```python
from build123d import *

# Parameters (mm, degrees)
SKETCH1_W           = 140
SKETCH1_H           = 93.753760253
BOSS_EXTRUDE1_DEPTH = 1.5
SKETCH2_R           = 1.6
CUT_EXTRUDE1_DEPTH  = 1.5
SKETCH3_R           = 2.737611944
SKETCH3_R_2         = 1.237611944
BOSS_EXTRUDE2_DEPTH = 8
SKETCH4_R           = 1.3
SKETCH4_R_2         = 1.35
SKETCH4_R_3         = 1.5875
CUT_EXTRUDE2_DEPTH  = 8


with BuildPart() as part:
    # Sketch1 → Boss-Extrude1 (new body)
    with BuildSketch(Plane.XY):
        with Locations((102, 196.095777869)):
            Rectangle(SKETCH1_W, SKETCH1_H)
    extrude(amount=BOSS_EXTRUDE1_DEPTH)

    # Sketch2 → Cut-Extrude1 (cut)
    with BuildSketch(Plane.XY.offset(1.5)):
        with Locations((47.04400772, 240.027868216)):
            Circle(SKETCH2_R)
        with Locations((162.04400772, 240.027868216)):
            Circle(SKETCH2_R)
    extrude(amount=-CUT_EXTRUDE1_DEPTH, mode=Mode.SUBTRACT)

    # Sketch3 → Boss-Extrude2 (add)
    # profile 1 of 2: a face of its own
    with BuildSketch(Plane.XY.offset(1.5)):
        with Locations((47.04400772, 156.027868216)):
            Circle(SKETCH3_R)
        with Locations((47.04400772, 156.027868216)):
            Circle(SKETCH3_R_2, mode=Mode.SUBTRACT)
    # profile 2 of 2: a face of its own
    with BuildSketch(Plane.XY.offset(1.5)):
        with Locations((162.04400772, 156.027868216)):
            Circle(SKETCH3_R)
        with Locations((162.04400772, 156.027868216)):
            Circle(SKETCH3_R_2, mode=Mode.SUBTRACT)
    extrude(amount=BOSS_EXTRUDE2_DEPTH)

    # Sketch4 → Cut-Extrude2 (cut)
    with BuildSketch(Plane(origin=(0, 0, 0), x_dir=(-1, 0, 0), z_dir=(0, 0, -1))):
        with Locations((-120.431826709, 209.617216317)):
            Circle(SKETCH4_R)
        with Locations((-62.434035172, 209.111077258)):
            Circle(SKETCH4_R_2)
        with Locations((-62.861635411, 160.112943028)):
            Circle(SKETCH4_R_2)
        with Locations((-120.859426949, 160.619082087)):
            Circle(SKETCH4_R_2)
        with Locations((-131.613133958, 181.551872542)):
            Circle(SKETCH4_R_3)
        with Locations((-136.693133958, 233.621872542)):
            Circle(SKETCH4_R_3)
        with Locations((-164.633133958, 233.621872542)):
            Circle(SKETCH4_R_3)
    extrude(amount=-CUT_EXTRUDE2_DEPTH, mode=Mode.SUBTRACT)


solid = part.part
```
Work out the finished part from the listing and answer in its coordinate system (mm). A direction names the side the tool comes from. Give positions to 0.01 mm unless a question says otherwise; leave off trailing zeros. Loops run counter-clockwise (first coordinate to the right, second up) from the corner with the lowest first, then second, coordinate; pieces in that order, holes last. Notation, with made-up numbers: M 47,48 L 52,48 A13 ccw 52,53 Z; hole C -32.5,-20.75 d6. An arc over 180 degrees is marked long. One line per item, written item: value. Start each with the question number.
1. Find the intervals of material crossed by probe 1 along Z at (x, y) = (111, 237); probe 2 along Y at (x, z) = (48, 6.75); probe 3 along X at (y, z) = (157.5, 8.25), in increasing order.
2. Determine the mould class of faces 3 (the face through (163, 155, 9.5)), 4 (the face through (132.783, 182.625, 0.74)) for opening direction X: released by +X, released by -X, zero draft, split by the parting line, or undercut.
3. Each of these flat-tipped pins is pushed along its axis until it touches: P1, Ø8, axis at x = 147.5, y = 211.5, coming from the +Z side; P2, Ø3, axis at x = 47.04, y = 156.03, coming from the -Z side. Where does it stop, or does it pass through?
4. Find section B-B (x = 110). Give the vertices of the cut face in (y, z).
5. Find section A-A (z = 5.5). Give the vertices of the cut face in (x, y), and give its area (3 significant figures).
6. Which of the six approach directions +Z, -Z, +X, -X, +Y, -Y give full straight-line access (tool end or side, diameter ignored) to faces 1 (the face through (160.774, 239.054, 0.76)), 2 (the face through (160.03, 157.88, 5.44))?
7. Find section C-C (y = 205.5). Give the vertices of the cut face in (x, z), and give its area (3 significant figures).
Reported:
1. probe 1: z = 0 to 1.5
1. probe 2: y = 153.46 to 155.24, 156.81 to 158.59
1. probe 3: x = 44.74 to 49.35, 159.74 to 164.35
2. face 3: zero draft
2. face 4: undercut
3. P1: stops at z = 1.5
3. P2: stops at z = 0
4. outline: M 149.22,0 L 242.97,0 L 242.97,1.5 L 149.22,1.5 Z
5. outline: C 47.04,156.03 d5.48; C 162.04,156.03 d5.48; hole C 47.04,156.03 d2.48; hole C 162.04,156.03 d2.48
5. area: 37.5 mm²
6. face 1: +Z, -Z
6. face 2: +Z
7. outline: M 32,0 L 172,0 L 172,1.5 L 32,1.5 Z
7. area: 210 mm²
